Can you work these out from the model? Positions are in its coordinate system, mm. Round coordinates to 2 decimals unless told otherwise and drop trailing zeros. Write each loop counter-clockwise with the first axis right and the second up, starting at its lowest first coordinate (ties: lowest second). Pieces come first, ordered by that corner, then holes. Notation, with made-up numbers: M 63.5,4 L 72.5,4 A25 ccw 72.5,26 Z; hole C 1,-8.5 d5. An arc over 180 degrees is marked long. Answer in a Markdown table with one row per item. Add a question column.
(1) Suppose I cut it at B-B, the plane z = 0.4. Count the separate pieces of the cut face and the enclosed holes in it, then the cut area to 3 significant figures.
(2) If I drill on probe 1 along X at (y, z) = (-0.5, 0.3); probe 2 along Y at (x, z) = (78.2, 0.65); probe 3 along Y at (x, z) = (-74.1, 0.7), over which ranges is the centre line in solid material (lowest first)?
(3) I'm going to push a flat-ended pin straight in: pin 1 (6.5 mm diameter, centred on x = 28.2, y = 9.5, fed in from -Z). Where does the tip first touch, or does it pass through?
(4) Suppose I cut it at A-A, the plane x = 8.2. Write out the boundary of the cut face in (y, z), then the cut area to 3 significant figures.
from build123d import *

# Parameters (mm, degrees)
SKETCH1_R           = 2.5
BOSS_EXTRUDE1_DEPTH = 1


with BuildPart() as part:
    # Sketch1 → Boss-Extrude1 (new body)
    with BuildSketch(Plane.XY):
        with BuildLine():
            ThreePointArc((-26.803847577, 33.5), (-29, 31.303847577), (-32, 30.5))
            ThreePointArc((-32, 30.5), (-35, 31.303847577), (-37.196152423, 33.5))
            Line((-37.196152423, 33.5), (-85, 33.5))
            Line((-85, 33.5), (-85, -33.5))
            Line((-85, -33.5), (85, -33.5))
            Line((85, -33.5), (85, 33.5))
            Line((85, 33.5), (-26.803847577, 33.5))
        make_face()
        with Locations((-68.3, -21.5)):
            Circle(SKETCH1_R, mode=Mode.SUBTRACT)
        with Locations((-74.1, 1.5)):
            Circle(SKETCH1_R, mode=Mode.SUBTRACT)
        with Locations((76.2, -22)):
            Circle(SKETCH1_R, mode=Mode.SUBTRACT)
        with Locations((18.7, -8.5)):
            Circle(SKETCH1_R, mode=Mode.SUBTRACT)
        with Locations((78.2, -0.1)):
            Circle(SKETCH1_R, mode=Mode.SUBTRACT)
        with Locations((-65.3, 20)):
            Circle(SKETCH1_R, mode=Mode.SUBTRACT)
        with Locations((8.2, 8.5)):
            Circle(SKETCH1_R, mode=Mode.SUBTRACT)
        with Locations((28.2, 9.5)):
            Circle(SKETCH1_R, mode=Mode.SUBTRACT)
        with Locations((73.2, 23.7)):
            Circle(SKETCH1_R, mode=Mode.SUBTRACT)
    extrude(amount=BOSS_EXTRUDE1_DEPTH)


solid = part.part
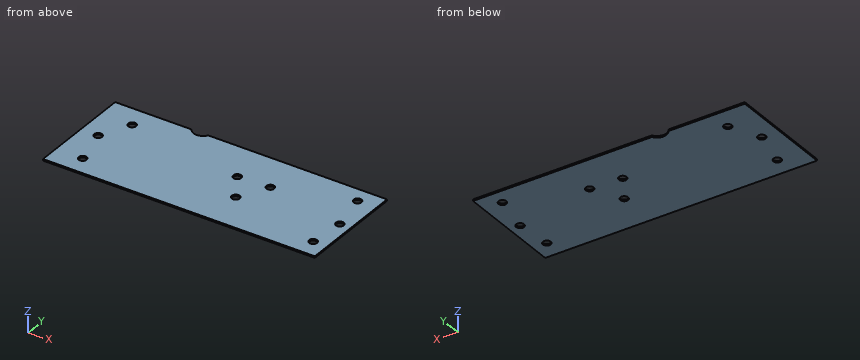
Calculated:
| question | item | result |
|---|---|---|
| 1 | separate pieces | 1 |
| 1 | enclosed holes | 9 |
| 1 | area | 11,200 mm² |
| 2 | probe 1 | -85 to -75.6, -72.6 to 75.73, 80.67 to 85 |
| 2 | probe 2 | -33.5 to -23.5, -20.5 to -2.6, 2.4 to 33.5 |
| 2 | probe 3 | -33.5 to -1, 4 to 33.5 |
| 3 | pin 1 | z = 0 |
| 4 | outline | M -33.5,0 L 6,0 L 6,1 L -33.5,1 Z; M 11,0 L 33.5,0 L 33.5,1 L 11,1 Z |
| 4 | area | 62.0 mm² |
